from build123d import *

# Parameters (mm, degrees)
BOSS_EXTRUDE2_DEPTH = 97.5
FILLET4_SIZE        = 3.6
SKETCH2_W           = 12.5
SKETCH2_H           = 4.91
CUT_EXTRUDE1_DEPTH  = 9.85
CUT_EXTRUDE2_DEPTH  = 10
SKETCH4_W           = 12.355512527
SKETCH4_H           = 2
BOSS_EXTRUDE3_DEPTH = 9


with BuildPart() as part:
    # Sketch1 → Boss-Extrude2 (new body)
    with BuildSketch(Plane.XY):
        Polygon((12.395, -11.5), (-12.395, -11.5), (-11.85, 11.5), (11.85, 11.5), align=None)
    extrude(amount=BOSS_EXTRUDE2_DEPTH)

    # Fillet4
    # a fillet whose section is not a circle: 3.6 mm, written as the material it takes off along each edge
    with BuildSketch(Plane(origin=(-12.608201023, -20.497474386, 0), x_dir=(0, 0, 1), z_dir=(0.023689002610023418, 0.9997193762028135, 0)), Plane(origin=(11.636798977, 20.497474386, 0), x_dir=(0, 0, 1), z_dir=(0.023689002610022953, -0.9997193762028134, 0))) as fillet4_piece_1:
        with BuildLine():
            add(Edge.make_bspline([(FILLET4_SIZE, 0), (FILLET4_SIZE * 0.831801948466, 0), (FILLET4_SIZE * 0.663603896932, 0), (FILLET4_SIZE * 0.292893218813, FILLET4_SIZE * 0.0716919198361), (FILLET4_SIZE * 0.0716919198361, FILLET4_SIZE * 0.292893218813), (0, FILLET4_SIZE * 0.663603896932), (0, FILLET4_SIZE * 0.831801948466), (0, FILLET4_SIZE)], knots=[0, 0, 0, 0, 0, 0, 0.5, 0.5, 1, 1, 1, 1, 1, 1], degree=5))
            Line((0, FILLET4_SIZE), (0, 0))
            Line((0, 0), (FILLET4_SIZE, 0))
        make_face()
    extrude(amount=41.006456159, mode=Mode.SUBTRACT)
    with BuildSketch(Plane(origin=(-12.608201023, -20.497474386, 97.5), x_dir=(0, 0, -1), z_dir=(0.023689002610023418, 0.9997193762028135, 0)), Plane(origin=(11.636798977, 20.497474386, 97.5), x_dir=(0, 0, -1), z_dir=(0.023689002610022953, -0.9997193762028134, 0))) as fillet4_piece_2:
        with BuildLine():
            add(Edge.make_bspline([(FILLET4_SIZE, 0), (FILLET4_SIZE * 0.831801948466, 0), (FILLET4_SIZE * 0.663603896932, 0), (FILLET4_SIZE * 0.292893218813, -FILLET4_SIZE * 0.0716919198361), (FILLET4_SIZE * 0.0716919198361, -FILLET4_SIZE * 0.292893218813), (0, -FILLET4_SIZE * 0.663603896932), (0, -FILLET4_SIZE * 0.831801948466), (0, -FILLET4_SIZE)], knots=[0, 0, 0, 0, 0, 0, 0.5, 0.5, 1, 1, 1, 1, 1, 1], degree=5))
            Line((0, -FILLET4_SIZE), (0, 0))
            Line((0, 0), (FILLET4_SIZE, 0))
        make_face()
    extrude(amount=41.006456159, mode=Mode.SUBTRACT)

    # Sketch2 → Cut-Extrude1 (cut)
    with BuildSketch(Plane.XY.offset(97.5)):
        with Locations((0, -2.845)):
            Rectangle(SKETCH2_W, SKETCH2_H)
    extrude(amount=-CUT_EXTRUDE1_DEPTH, mode=Mode.SUBTRACT)

    # Sketch3 → Cut-Extrude2 (cut)
    with BuildSketch(Plane.XY.offset(97.5)):
        with BuildLine():
            Line((-3.629235437, 2.994588956), (-2.719235437, 2.5506273))
            ThreePointArc((-2.719235437, 2.5506273), (-2.612502556, 2.512821208), (-2.5, 2.5))
            Line((-2.5, 2.5), (2.5, 2.5))
            ThreePointArc((2.5, 2.5), (2.612502556, 2.512821208), (2.719235437, 2.5506273))
            Line((2.719235437, 2.5506273), (3.629235437, 2.994588956))
            ThreePointArc((3.629235437, 2.994588956), (3.834038747, 3.179025548), (3.91, 3.443961655))
            Line((3.91, 3.443961655), (3.91, 4.7))
            ThreePointArc((3.91, 4.7), (3.763553391, 5.053553391), (3.41, 5.2))
            Line((3.41, 5.2), (-3.41, 5.2))
            ThreePointArc((-3.41, 5.2), (-3.763553391, 5.053553391), (-3.91, 4.7))
            Line((-3.91, 4.7), (-3.91, 3.443961655))
            ThreePointArc((-3.91, 3.443961655), (-3.834038747, 3.179025548), (-3.629235437, 2.994588956))
        make_face()
    extrude(amount=-CUT_EXTRUDE2_DEPTH, mode=Mode.SUBTRACT)

    # Sketch4 → Boss-Extrude3 (add)
    with BuildSketch(Plane.XY.offset(87.65)):
        with Locations((0.018279413, -4.198858777)):
            Rectangle(SKETCH4_W, SKETCH4_H)
    extrude(amount=BOSS_EXTRUDE3_DEPTH)


solid = part.part
Here's how the part is built. I have some questions about the finished solid (model axes, mm). A direction names the side the tool comes from. Coordinates: 2 decimals unless noted, no trailing zeros. Write each loop counter-clockwise with the first axis right and the second up, starting at its lowest first coordinate (ties: lowest second). Pieces come first, ordered by that corner, then holes.
Item 1: Will these pins go through, and if not, where does the flat tip stop? pin 1 (1 mm diameter, centred on y = -4, z = 93, fed in from -X); pin 2 (4 mm diameter, centred on y = -4, z = 92.5, fed in from -X); pin 3 (1.4 mm diameter, centred on y = 4, z = 94, fed in from -X).
Item 2: I want a section at B-B on z = 53.5. Write out the boundary of the cut face in (x, y) (3 decimals).
Item 3: If we mould it in two halves opening along X, with no side actions, what happens to faces 3 (the flat face through (0, 11.5, 48)), 4 (the flat face through (0, 4, 87.5))? For each: +X half, -X half, draft (parallel to the pull), parting line (faces both ways), or undercut.
Item 4: On a 3-axis mill with a long thin cutter (end or side, diameter ignored), from which of +Z, -Z, +X, -X, +Y, -Y can I reach the whole of each face in a straight line? I mean faces 1 (the flat face through (0, -0.39, 93)), 2 (the flat face through (0, 0, 0)). Say none if no direction works.
Item 5: I want a section at A-A on x = -0.5. Write out the boundary of the cut face in (y, z).
Item 6: If I drill on line 1 (X direction, y = 10.75, z = 79.5); line 2 (Z direction, x = 10.5, y = 9.5); line 3 (X direction, y = -3.5, z = 75.5), over which ranges is the centre line in solid material (lowest first)?
Findings below:
1. pin 1: stops at x = -12.23
1. pin 2: stops at x = -12.26
1. pin 3: stops at x = -12.04
2. outline: (-12.395, -11.5) - (12.395, -11.5) - (11.85, 11.5) - (-11.85, 11.5) - close
3. face 3: draft
3. face 4: undercut
4. face 1: +Z
4. face 2: -Z, +X, -X, +Y, -Y
5. outline: (-11.5, 0) - (11.5, 0) - (11.5, 97.5) - (5.2, 97.5) - (5.2, 87.5) - (2.5, 87.5) - (2.5, 97.5) - (-0.39, 97.5) - (-0.39, 87.65) - (-3.2, 87.65) - (-3.2, 96.65) - (-5.2, 96.65) - (-5.2, 87.65) - (-5.3, 87.65) - (-5.3, 97.5) - (-11.5, 97.5) - close
6. line 1: x = -11.87 to 11.87
6. line 2: z = 0.36 to 97.14
6. line 3: x = -12.21 to 12.21
